Geometry check sheet. Reference: the model listing, model coordinates, mm. A direction names the side the tool comes from. Round coordinates to 2 decimals unless told otherwise and drop trailing zeros. Write each loop counter-clockwise with the first axis right and the second up, starting at its lowest first coordinate (ties: lowest second). Pieces come first, ordered by that corner, then holes.
from build123d import *

# Parameters (mm, degrees)
SKETCH1_W           = 170
SKETCH1_H           = 7.8
BOSS_EXTRUDE1_DEPTH = 7.8
SKETCH2_W           = 20
SKETCH2_H           = 7.8
BOSS_EXTRUDE2_DEPTH = 71
SKETCH3_R           = 3.9
BOSS_EXTRUDE3_DEPTH = 43
SKETCH4_W           = 20
SKETCH4_H           = 7.8
BOSS_EXTRUDE4_DEPTH = 25
SKETCH5_W           = 10
SKETCH5_H           = 7.8
CUT_EXTRUDE1_DEPTH  = 119.646151442
SKETCH6_W           = 5
SKETCH6_H           = 7.8
BOSS_EXTRUDE5_DEPTH = 5


with BuildPart() as part:
    # Sketch1 → Boss-Extrude1 (new body)
    with BuildSketch(Plane(origin=(0, 0, 0), x_dir=(1, 0, 0), z_dir=(0, 1, 0))):
        with Locations((9.736842105, 9.155198973)):
            Rectangle(SKETCH1_W, SKETCH1_H)
    extrude(amount=BOSS_EXTRUDE1_DEPTH)

    # Sketch2 → Boss-Extrude2 (add)
    with BuildSketch(Plane.XY.offset(-5.255198973)):
        with Locations((-20.263157895, 3.9)):
            Rectangle(SKETCH2_W, SKETCH2_H)
    boss_extrude2 = extrude(amount=BOSS_EXTRUDE2_DEPTH)

    # Sketch3 → Boss-Extrude3 (add)
    with BuildSketch(Plane.ZY.offset(30.263157895)):
        with Locations((61.844801027, 3.9)):
            Circle(SKETCH3_R)
    boss_extrude3 = extrude(amount=BOSS_EXTRUDE3_DEPTH)

    # Sketch4 → Boss-Extrude4 (add)
    with BuildSketch(Plane(origin=(-10.263157895, 0, 0), x_dir=(0, 0, -1), z_dir=(1, 0, 0))):
        with Locations((-55.744801027, 3.9)):
            Rectangle(SKETCH4_W, SKETCH4_H)
    boss_extrude4 = extrude(amount=BOSS_EXTRUDE4_DEPTH)

    # Mirror1: Boss-Extrude2, Boss-Extrude3, Boss-Extrude4 across plane
    add(boss_extrude2.mirror(Plane.ZY.offset(-9.736842105)))
    add(boss_extrude3.mirror(Plane.ZY.offset(-9.736842105)))
    add(boss_extrude4.mirror(Plane.ZY.offset(-9.736842105)))

    # Sketch5 → Cut-Extrude1 (cut, through all)
    with BuildSketch(Plane.XY.offset(-5.255198973)):
        with Locations((19.736842105, 3.9)):
            Rectangle(SKETCH5_W, SKETCH5_H)
    extrude(amount=-CUT_EXTRUDE1_DEPTH, mode=Mode.SUBTRACT)

    # Sketch6 → Boss-Extrude5 (add)
    with BuildSketch(Plane.XY.offset(-5.255198973)):
        with Locations((-2.763157895, 3.9)):
            Rectangle(SKETCH6_W, SKETCH6_H)
    extrude(amount=BOSS_EXTRUDE5_DEPTH)


solid = part.part
1. Depth check by flat-ended pin: pin 1 Ø2 at (x, y) = (51.5, 6.5) entering from +Z; pin 2 Ø1.5 at (y, z) = (4.5, -3.5) entering from +X; pin 3 Ø3 at (x, y) = (52.5, 2) entering from +Z; pin 4 Ø6 at (x, z) = (-5, 55) entering from -Y. Enter the tip coordinate at first touch or a pass-through.
2. Section check D-D (y = 2.5). Record the cut outline in (x, z), plus the area to 3 significant figures.
3. Release check for a two-part mould opening along X. For faces 1 (the face through (30, 0, 27)), 2 (the face through (-0.263, 4, -3)), 3 (the face through (-30.263, 4, 28)) record: +X half, -X half, draft (parallel to the pull), parting line (faces both ways), or undercut.
4. Section check B-B (z = -3). Record the cut outline in (x, y), plus the area to 3 significant figures.
5. Section check A-A (x = 6.5). Record the cut outline in (y, z).
6. Section check C-C (z = 43). Record the cut outline in (x, y).
7. Scan lines: line 1 along X through (y, z) = (6.5, -5); line 2 along Z through (x, y) = (85, 3.5); line 3 along X through (y, z) = (1.5, 22.5). Record each from-to range of solid material in increasing order.
8. Access from +Z, -Z, +X, -X, +Y, -Y to the whole of each face (thin tool, end or side, straight path). Record for faces 4 (the face through (-10.263, 4, 20)), 5 (the face through (14.737, 4, -9)), 6 (the face through (-53, 4, -5.255)), 7 (the face through (-30.263, 1, 65)).
Results below:
1. pin 1: stops at z = 65.4
1. pin 2: stops at x = 49.74
1. pin 3: stops at z = 65.72
1. pin 4: stops at y = 0
2. outline: (-75.26, -13.06) - (14.74, -13.06) - (14.74, -5.26) - (-0.26, -5.26) - (-0.26, -0.26) - (-5.26, -0.26) - (-5.26, -5.26) - (-10.26, -5.26) - (-10.26, 45.74) - (29.74, 45.74) - (29.74, -5.26) - (24.74, -5.26) - (24.74, -13.06) - (94.74, -13.06) - (94.74, -5.26) - (49.74, -5.26) - (49.74, 58.2) - (92.74, 58.2) - (92.74, 65.48) - (49.74, 65.48) - (49.74, 65.74) - (-30.26, 65.74) - (-30.26, 65.48) - (-73.26, 65.48) - (-73.26, 58.2) - (-30.26, 58.2) - (-30.26, -5.26) - (-75.26, -5.26) - close
2. area: 5,540 mm2
3. face 1: draft
3. face 2: undercut
3. face 3: -X half
4. outline: (-30.26, 0) - (-10.26, 0) - (-10.26, 7.8) - (-30.26, 7.8) - close; (-5.26, 0) - (-0.26, 0) - (-0.26, 7.8) - (-5.26, 7.8) - close; (29.74, 0) - (49.74, 0) - (49.74, 7.8) - (29.74, 7.8) - close
4. area: 351 mm2
5. outline: (0, -13.06) - (7.8, -13.06) - (7.8, -5.26) - (0, -5.26) - close; (0, 45.74) - (7.8, 45.74) - (7.8, 65.74) - (0, 65.74) - close
6. outline: (-30.26, 0) - (-10.26, 0) - (-10.26, 7.8) - (-30.26, 7.8) - close; (29.74, 0) - (49.74, 0) - (49.74, 7.8) - (29.74, 7.8) - close
7. line 1: x = -30.26 to -10.26, -5.26 to -0.26, 29.74 to 49.74
7. line 2: z = -13.06 to -5.26, 57.97 to 65.72
7. line 3: x = -30.26 to -10.26, 29.74 to 49.74
8. face 4: +Y, -Y
8. face 5: -Z, +Y, -Y
8. face 6: -X, +Y, -Y
8. face 7: +Z, -X, -Y
